Part model, mm, in its own coordinate system. A direction names the side the tool comes from. Coordinates: 2 decimals unless noted, no trailing zeros. Write each loop counter-clockwise with the first axis right and the second up, starting at its lowest first coordinate (ties: lowest second). Pieces come first, ordered by that corner, then holes. Notation, with made-up numbers: (23, 22) - (34, 22) arc R13 cw to (34, 33) - close; hole circle Ø5 at (52, 73.25). An arc over 180 degrees is marked (long way). Use one line per item in the form item = value. Start each with the question number.
from build123d import *

# Parameters (mm, degrees)
IZIM3_R                     = 1.5
Y_KSEKLIK_EKSTR_ZYON1_DEPTH = 3


with BuildPart() as part:
    # Çizim3 → Yükseklik-Ekstrüzyon1 (new body)
    with BuildSketch(Plane.XY):
        with BuildLine():
            ThreePointArc((-21.522830549, 9.375995553), (-34.375995553, 3.477169451), (-28.477169451, -9.375995553))
            ThreePointArc((-28.477169451, -9.375995553), (-0.585261649, -14.367996391), (27.297293596, -9.324019171))
            ThreePointArc((27.297293596, -9.324019171), (33.172153672, 3.540117765), (20.308016736, 9.41497784))
            ThreePointArc((20.308016736, 9.41497784), (-0.603899698, 5.631994925), (-21.522830549, 9.375995553))
        make_face()
        with Locations((-25, 0)):
            Circle(IZIM3_R, mode=Mode.SUBTRACT)
        with Locations((-25, 5)):
            Circle(IZIM3_R, mode=Mode.SUBTRACT)
        with Locations((-30, 0)):
            Circle(IZIM3_R, mode=Mode.SUBTRACT)
        with Locations((-20, 0)):
            Circle(IZIM3_R, mode=Mode.SUBTRACT)
        with Locations((-25, -5)):
            Circle(IZIM3_R, mode=Mode.SUBTRACT)
        with Locations((23.802655166, 0.045479334)):
            Circle(IZIM3_R, mode=Mode.SUBTRACT)
        with Locations((23.802655166, 5.045479334)):
            Circle(IZIM3_R, mode=Mode.SUBTRACT)
        with Locations((28.802448325, 0)):
            Circle(IZIM3_R, mode=Mode.SUBTRACT)
        with Locations((18.802655166, 0.045479334)):
            Circle(IZIM3_R, mode=Mode.SUBTRACT)
        with Locations((23.802655166, -4.954520666)):
            Circle(IZIM3_R, mode=Mode.SUBTRACT)
        with BuildLine():
            ThreePointArc((-9.420289855, 0.673684705), (0, -0.012567627), (9.420289855, 0.673684705))
            ThreePointArc((9.420289855, 0.673684705), (13.957769087, -2.704374237), (10.579710145, -7.241853469))
            ThreePointArc((10.579710145, -7.241853469), (0, -8.012567627), (-10.579710145, -7.241853469))
            ThreePointArc((-10.579710145, -7.241853469), (-13.957769087, -2.704374237), (-9.420289855, 0.673684705))
        make_face(mode=Mode.SUBTRACT)
    extrude(amount=Y_KSEKLIK_EKSTR_ZYON1_DEPTH)


solid = part.part
Q1. Pin check, flat tips, straight feed: P1, Ø2.5, axis at x = -20, y = 0, coming from the -Z side; P2, Ø5, axis at x = -30, y = 0, coming from the -Z side; P3, Ø1, axis at x = 2, z = 1, coming from the +Y side. Stop position of each tip, or through.
Q2. Which spindle directions (+Z, -Z, +X, -X, +Y, -Y) get a long thin tool onto all of the face, cutting with end or side? Do faces 1 (the cylindrical face through (-0.132, -0.012, 1.479)), 2 (the flat face through (-1, 1, 3)). Say none if no direction does.
Q3. Drill centre lines: probe 1 along Y at (x, z) = (-25, 0.8); probe 2 along X at (y, z) = (-4, 2.5); probe 3 along Y at (x, z) = (-1.5, 2.4). Where is each one in solid material? Low to high.
Q4. Slice it at C-C (x = 29). List the corners of the cut face in (y, z), plus the area to 3 significant figures.
Q5. Slice it at A-A (x = -25). List the corners of the cut face in (y, z), plus the area to 3 significant figures.
Q6. Slice it at B-B (y = 8.25). List the corners of the cut face in (x, z).
Q7. Mould opens along Y. For faces 3 (the cylindrical face through (13.944, -2.617, 1.479)), 4 (the cylindrical face through (-26.5, 0.07, 1.48)), 5 (the cylindrical face through (-0.984, -14.367, 1.479)), 6 (the cylindrical face through (-0.305, 5.633, 1.479)) say: released by +Y, released by -Y, zero draft, split by the parting line, or undercut.
Q8. Slice it at D-D (z = 1.7). Count the separate pieces of the cut face and the enclosed holes in it, plus the area to 3 significant figures.
Solution:
q1.P1 = through
q1.P2 = 0
q1.P3 = 5.72
q2.face_1 = +Z, -Z
q2.face_2 = +Z, +X, -X, +Y, -Y
q3.probe_1 = -10.58 to -6.5, -3.5 to -1.5, 1.5 to 3.5, 6.5 to 10
q3.probe_2 = -34.17 to -26.12, -23.88 to -13.94, 13.94 to 22.65, 24.96 to 32.95
q3.probe_3 = -14.36 to -8, 0 to 5.64
q4.outline = (-8.5, 0) - (-1.49, 0) - (-1.49, 3) - (-8.5, 3) - close; (1.49, 0) - (8.59, 0) - (8.59, 3) - (1.49, 3) - close
q4.area = 42.3 mm2
q5.outline = (-10.58, 0) - (-6.5, 0) - (-6.5, 3) - (-10.58, 3) - close; (-3.5, 0) - (-1.5, 0) - (-1.5, 3) - (-3.5, 3) - close; (1.5, 0) - (3.5, 0) - (3.5, 3) - (1.5, 3) - close; (6.5, 0) - (10, 0) - (10, 3) - (6.5, 3) - close
q5.area = 34.7 mm2
q6.outline = (-30.65, 0) - (-18.19, 0) - (-18.19, 3) - (-30.65, 3) - close; (16.87, 0) - (29.52, 0) - (29.52, 3) - (16.87, 3) - close
q7.face_3 = undercut
q7.face_4 = undercut
q7.face_5 = released by -Y
q7.face_6 = released by +Y
q8.separate_pieces = 1
q8.enclosed_holes = 11
q8.area = 1,030 mm2
